Design review of the part built by this model. Coordinates are the model's own, in mm. A direction names the side the tool comes from. Round coordinates to 2 decimals unless told otherwise and drop trailing zeros. Order: outer loops, then holes, each group sorted by start corner. A loop starts at its lowest first (then second) coordinate and runs counter-clockwise, first axis right, second up. Notation, with made-up numbers: M 30,38.5 L 75,38.5 A24 ccw 75,51.5 Z; hole C 66,33 d4. An arc over 180 degrees is marked long. Write item = value, one per line. Start each with the question number.
Autodesk Inventor part; units mm, degrees
ref_plane "YZ Plane" through (0, 0, 0) normal (1, 0, 0) x (0, 1, 0)
ref_plane "XZ Plane" through (0, 0, 0) normal (0, 1, 0) x (-1, 0, 0)
ref_plane "XY Plane" through (0, 0, 0) normal (0, 0, 1) x (1, 0, 0)
sketch "Sketch1" plane through (0, 0, 0) normal (0, 1, 0) x (-1, 0, 0)
  circle A0 centre (0, 0) radius 13.55
  dimension "d0" = 27.1
extrude "Extrusion1" add sketch "Sketch1" along normal blind 4.15
sketch "Sketch2" plane through (0, 4.15, 0) normal (0, 1, 0) x (1, 0, 0)
  circle A0 centre (0, 0) radius 10.1625
  dimension "d3" = 20.325
extrude "Extrusion2" add sketch "Sketch2" along normal blind 4.15
fillet "Fillet1" radius 3.175 1 edges at (-10.1625, 8.3, 0)
fillet "Fillet2" radius 3.175 1 edges at (13.55, 4.15, 0)
sketch "Sketch3" plane through (0, 0, 0) normal (0, -1, 0) x (1, 0, 0)
  circle A0 centre (0, 0) radius 11.75
  dimension "d8" = 23.5
extrude "Extrusion3" add sketch "Sketch3" along normal blind 24.7
properties part number "small_button"
(1) Insertion check: pin 1 (4 mm diameter, centred on x = -6.5, y = 3.5, fed in from +Z); pin 2 (8 mm diameter, centred on y = -13, z = -10.5, fed in from +X); pin 3 (1.5 mm diameter, centred on y = -6, z = -3.5, fed in from +X). Each pin has a flat end and moves straight along its axis. Give the tip position at first contact, or say it passes through.
(2) Consider section C-C, the plane y = -22. Write out the cut boundary in (x, z).
(3) For faces 1 (the face through (9.693, 4.631, 3.053)), 2 (the face through (0, -24.7, 0)), 3 (the face through (0, 0, 12)), list the 3-axis set-ups (+Z, -Z, +X, -X, +Y, -Y) from which the entire face can be reached by the end or side of a thin tool; tool diameter is ignored.
(4) For line 1 along Z through (x, y) = (-2.75, -6.5); line 2 along X through (y, z) = (-6, 8); line 3 along X through (y, z) = (1, 9.5), list the stretches that pass through material, from the lowest coordinate up. Write a range as [from, to].
Completed:
q1.pin_1 = 12.34
q1.pin_2 = 9.79
q1.pin_3 = 11.42
q2.outline = C 0,0 d23.5
q3.face_1 = +Y
q3.face_2 = +Z, -Z, +X, -X, -Y
q3.face_3 = -Y
q4.line_1 = [-11.42, 11.42]
q4.line_2 = [-8.61, 8.61]
q4.line_3 = [-9.66, 9.66]
